Can you work these out from the model? Positions are in its coordinate system, mm. Face numbers are marked on the shaded views. Coordinates: 2 decimals unless noted, no trailing zeros. Order: outer loops, then holes, each group sorted by start corner. A loop starts at its lowest first (then second) coordinate and runs counter-clockwise, first axis right, second up. Notation, with made-up numbers: (55, 86.25) -> (62, 86.25) arc R34 ccw to (62, 123.25) -> close; hole circle Ø3 at (-10, 61). An arc over 180 degrees is marked (long way). Return JSON: item names as keys, results as strings. Group by question number.
1) If we section it at A-A, the plane y = 3.75: Please give me the cut outline in (x, z), then the cut area to 3 significant figures.
2) If we section it at D-D, the plane y = 2: Please give me the cut outline in (x, z).
3) If we section it at C-C, the plane x = 0: Please give me the cut outline in (y, z), then the cut area to 3 significant figures.
4) Thinking about a two-plate mould opening in Z: for the marked faces 1, 2 and 3, which applies, +Z half, -Z half, draft (parallel to the pull), parting line (faces both ways), or undercut?
5) For pin 1 (1.5 mm diameter, centred on x = -4, z = -3, fed in from +Y); pin 2 (1.8 mm diameter, centred on x = -1, z = -3, fed in from +Y); pin 3 (1 mm diameter, centred on y = 7, z = 1, fed in from -X), each with a flat end and sliding along its axis, tell me the tip position at first contact or that it passes through.
6) If I drill on probe 1 along X at (y, z) = (3.75, -4.5); probe 2 along X at (y, z) = (3.75, -3.75); probe 3 along Z at (x, y) = (0, 7.25), over which ranges is the centre line in solid material (lowest first)? Write a range as from..to.
7) If we section it at B-B, the plane z = -2.1: Please give me the cut outline in (x, y).
Autodesk Inventor part; units mm, degrees
ref_plane "YZ Plane" through (0, 0, 0) normal (1, 0, 0) x (0, 1, 0)
ref_plane "XZ Plane" through (0, 0, 0) normal (0, 1, 0) x (-1, 0, 0)
ref_plane "XY Plane" through (0, 0, 0) normal (0, 0, 1) x (1, 0, 0)
sketch "Sketch1" plane through (0, 0, 0) normal (0, 1, 0) x (-1, 0, 0)
  line L0 (0, 0) -> (0, -4.2)
  circle A0 centre (0, -2.1) radius 2.1
  line L1 (0, -2.1) -> (0, -6.9)
  line L2 (0, -6.9) -> (0, 2.7)
  line L3 (0, 2.7) -> (5, 2.7)
  line L4 (5, 2.7) -> (5, -7.3)
  line L5 (5, -7.3) -> (-5, -7.3)
  line L6 (-5, -7.3) -> (-5, 2.7)
  line L7 (-5, 2.7) -> (0, 2.7)
  dimension "d0" = 4.2
  dimension "d1" = 4.8
  dimension "d2" = 9.6
  dimension "d3" = 5
  dimension "d4" = 10
extrude "Extrusion1" add sketch "Sketch1" along normal blind 10
sketch "Sketch2" plane through (0, 10, 0) normal (0, 1, 0) x (1, 0, 0)
  circle A0 centre (0, 2.1) radius 2.1
  circle A1 centre (0, 2.1) radius 3
  point P0 (0, 0)
  dimension "d7" = 6
extrude "Extrusion2" cut sketch "Sketch2" against normal blind 3.5 contours A0 | A1
fillet "Fillet1" radius 5 2 edges at (5, 10, -2.3) (-5, 10, -2.3)
sketch "Sketch3" plane through (-5, 0, 2.7) normal (0, 0, 1) x (1, 0, 0)
  arc A0 (10, 5) -> (0, 5) centre (5, 5) ccw
  line L0 (5, 5) -> (5, 10)
  line L1 (5, 5) -> (5, 0)
  line L2 (5, 0) -> (5, 5)
  line L3 (0, 0) -> (0, 5)
  line L4 (5, 5) -> (0, 5)
  line L5 (0, 5) -> (2.5, 5)
  line L6 (2.5, 5) -> (2.5, 0)
  line L7 (2.5, 0) -> (2.5, 2.5)
  line L8 (1.25, 5) -> (1.25, 0)
  line L9 (0, 0) -> (10, 0)
  line L10 (2.5, 2.5) -> (1.25, 2.5)
  line L11 (1.875, 5) -> (1.875, 2.5)
  circle A1 centre (1.875, 2.5) radius 1.15
  line L12 (1.25, 5) -> (1.875, 5)
  line L13 (1.5625, 5) -> (1.5625, 2.5)
  line L14 (1.5625, 2.5) -> (1.5625, 3.75)
  circle A2 centre (1.5625, 3.75) radius 1.15
  line L15 (1.5625, 3.75) -> (0.4125, 3.75)
  line L16 (0.4125, 3.75) -> (0, 3.75)
  dimension "d14" = 2.3
extrude "Extrusion3" cut sketch "Sketch3" against normal through all contours L15 L8 A1 A2 | A2 L8 L15 | A2 L13 L15 L8 | A2 A1 L6 | L6 A1 L11 A2 | A1 L8 A2 | L15 L13 A1 L8 | A2 L11 A1 L13 | A1 A2 L6 | L6 A2 L11 A1 | A1 L13 A2 L8 | L11 A2 L13 A1 picked at (2.5388, 4.0306) picked at (1.186, 3.1393) picked at (2.5186, 3.2399)
properties part number "pist"
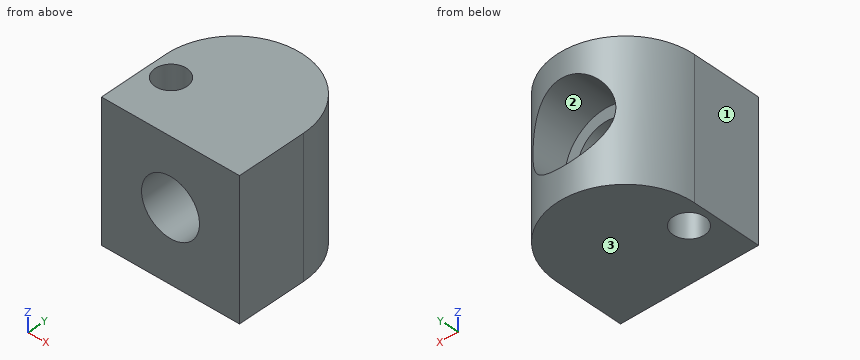
Result sheet:
{
 "1": {"outline": "(-5, -7.3) -> (-4.59, -7.3) -> (-4.59, 2.7) -> (-5, 2.7) -> close; (-2.29, -7.3) -> (5, -7.3) -> (5, 2.7) -> (-2.29, 2.7) -> close; hole circle Ø4.2 at (0, -2.1)", "area": "63.1 mm2"},
 "2": {"outline": "(-5, -7.3) -> (5, -7.3) -> (5, 2.7) -> (-5, 2.7) -> close; hole circle Ø4.2 at (0, -2.1)"},
 "3": {"outline": "(0, -7.3) -> (10, -7.3) -> (10, -5.1) -> (6.5, -5.1) -> (6.5, -4.2) -> (0, -4.2) -> close; (0, 0) -> (6.5, 0) -> (6.5, 0.9) -> (10, 0.9) -> (10, 2.7) -> (0, 2.7) -> close", "area": "51.7 mm2"},
 "4": {"face 1": "draft", "face 2": "undercut", "face 3": "-Z half"},
 "5": {"pin 1": "stops at y = 8.8", "pin 2": "stops at y = 6.5", "pin 3": "stops at x = -4.77"},
 "6": {"probe 1": "x = -5..-4.59, -2.29..5", "probe 2": "x = -5..-4.59, -2.29..-1.3, 1.3..5", "probe 3": "z = -7.3..-5.1, 0.9..2.7"},
 "7": {"outline": "(-5, 0) -> (-2.1, 0) -> (-2.1, 6.5) -> (-3, 6.5) -> (-3, 9) arc R5 ccw to (-5, 5) -> close; (2.1, 0) -> (5, 0) -> (5, 5) arc R5 ccw to (3, 9) -> (3, 6.5) -> (2.1, 6.5) -> close; hole circle Ø2.3 at (-3.44, 3.75)"}
}
